from build123d import *

# Parameters (mm, degrees)
F0_W      = 114.3
F0_H      = 50.8
F1_DEPTH  = 12.7
F2_R      = 3.175
F3_DEPTH  = 38.1
F4_R      = 3.175
F5_DEPTH  = 6.35
F6_R      = 38.1
F7_DEPTH  = 12.7
F9_R      = 19.05
F10_DEPTH = 0.8128
F11_R     = 3.175
F12_DEPTH = 12.7


with BuildPart() as f1:
    # F0 (on Right) → F1 (new body, symmetric)
    with BuildSketch(Plane.YZ):
        Rectangle(F0_W, F0_H)
    extrude(amount=F1_DEPTH, both=True)

    # F2 (on face) → F3 (join)
    with BuildSketch(Plane(origin=(0, 0, -25.4), x_dir=(1, 0, 0), z_dir=(0, 0, -1))):
        Circle(F2_R)
    extrude(amount=F3_DEPTH)

    # F4 (on face) → F5 (join)
    with BuildSketch(Plane.YZ.offset(12.7)):
        with Locations((-44.45, 0)):
            Circle(F4_R)
        with Locations((44.45, 0)):
            Circle(F4_R)
    extrude(amount=F5_DEPTH)

    # F6 (on face) → F7 (join)
    with BuildSketch(Plane.YZ.offset(19.05)):
        with Locations((-44.45, 0)):
            Circle(F6_R)
        with Locations((44.45, 0)):
            Circle(F6_R)
    extrude(amount=F7_DEPTH)

    # F8: F1 across plane


with BuildPart() as f1_1:
    add(f1.part)
    add(f1.part.mirror(Plane.YZ))

    # F9 (on face) → F10 (join)
    with BuildSketch(Plane(origin=(0, 0, -63.5), x_dir=(1, 0, 0), z_dir=(0, 0, -1))):
        Circle(F9_R)
    extrude(amount=F10_DEPTH)

    # F11 (on face) → F12 (join)
    with BuildSketch(Plane(origin=(0, 0, -64.3128), x_dir=(1, 0, 0), z_dir=(0, 0, -1))):
        Circle(F11_R)
    extrude(amount=F12_DEPTH)


solid = f1_1.part
Verification items for the finished model (mm, model axes). A direction names the side the tool comes from. Coordinates: 2 decimals unless noted, no trailing zeros. Write each loop counter-clockwise with the first axis right and the second up, starting at its lowest first coordinate (ties: lowest second). Pieces come first, ordered by that corner, then holes. Notation, with made-up numbers: M 33.5,54 L 46.5,54 A23 ccw 46.5,75 Z; hole C -20,-35.5 d1. An arc over 180 degrees is marked long. One line per question, with ' | ' between items.
1) Material ranges on L1, parallel to X at y = 24, z = -20; L2, parallel to X at y = 73.5, z = -7; L3, parallel to Z at x = 11, y = -12.5, recorded low to high.
Solutions:
L1: -31.75 to -19.05, -12.7 to 12.7, 19.05 to 31.75 | L2: -31.75 to -19.05, 19.05 to 31.75 | L3: -64.31 to -63.5, -25.4 to 25.4
2) Depth check by flat-ended pin: pin 1 Ø10 at (x, y) = (-17.5, -62) entering from -Z; pin 2 Ø6 at (x, z) = (6.5, -8) entering from -Y; pin 3 Ø4 at (x, z) = (2.5, -36) entering from -Y. Enter the tip coordinate at first touch or a pass-through.
Solutions:
pin 1: z = -35.89 | pin 2: y = -57.15 | pin 3: y = -3.14
3) Access from +Z, -Z, +X, -X, +Y, -Y to the whole of each face (thin tool, end or side, straight path). Record for faces 1 (the face through (15.83, -41.42, 0.95)), 2 (the face through (-25.31, 80.79, 11.44)), 3 (the face through (-15.12, 11.59, -63.9)), 4 (the face through (0, -57.15, 0)).
Solutions:
face 1: none | face 2: -X | face 3: -Z | face 4: +Z, -Z, -Y
4) Sectioned sample at A-A on z = 12. Record the cut outline in (x, y).
Solutions:
outline: M -31.75,-80.61 L -19.05,-80.61 L -19.05,-8.29 L -31.75,-8.29 Z; M -31.75,8.29 L -19.05,8.29 L -19.05,80.61 L -31.75,80.61 Z; M -12.7,-57.15 L 12.7,-57.15 L 12.7,57.15 L -12.7,57.15 Z; M 19.05,-80.61 L 31.75,-80.61 L 31.75,-8.29 L 19.05,-8.29 Z; M 19.05,8.29 L 31.75,8.29 L 31.75,80.61 L 19.05,80.61 Z
5) Sectioned sample at C-C on x = 0. Record the cut outline in (y, z) (3 decimals), then the cut area to 3 significant figures.
Solutions:
outline: M -57.15,-25.4 L -3.175,-25.4 L -3.175,-63.5 L -19.05,-63.5 L -19.05,-64.313 L -3.175,-64.313 L -3.175,-77.013 L 3.175,-77.013 L 3.175,-64.313 L 19.05,-64.313 L 19.05,-63.5 L 3.175,-63.5 L 3.175,-25.4 L 57.15,-25.4 L 57.15,25.4 L -57.15,25.4 Z | area: 6,160 mm^2
6) Sectioned sample at D-D on y = 31. Record the cut outline in (x, z).
Solutions:
outline: M -31.75,-35.65 L -19.05,-35.65 L -19.05,35.65 L -31.75,35.65 Z; M -12.7,-25.4 L 12.7,-25.4 L 12.7,25.4 L -12.7,25.4 Z; M 19.05,-35.65 L 31.75,-35.65 L 31.75,35.65 L 19.05,35.65 Z
7) Release check for a two-part mould opening along Z. For faces 5 (the face through (-15.83, 41.28, 0.14)), 6 (the face through (-12.7, -1, 0)), 7 (the face through (-0.69, 3.1, -44.18)) record: +Z half, -Z half, draft (parallel to the pull), parting line (faces both ways), or undercut.
Solutions:
face 5: parting line | face 6: draft | face 7: undercut
8) Sectioned sample at B-B on y = 0. Record the cut outline in (x, z) (3 decimals), then the cut area to 3 significant figures.
Solutions:
outline: M -19.05,-64.313 L -3.175,-64.313 L -3.175,-77.013 L 3.175,-77.013 L 3.175,-64.313 L 19.05,-64.313 L 19.05,-63.5 L 3.175,-63.5 L 3.175,-25.4 L 12.7,-25.4 L 12.7,25.4 L -12.7,25.4 L -12.7,-25.4 L -3.175,-25.4 L -3.175,-63.5 L -19.05,-63.5 Z | area: 1,640 mm^2
